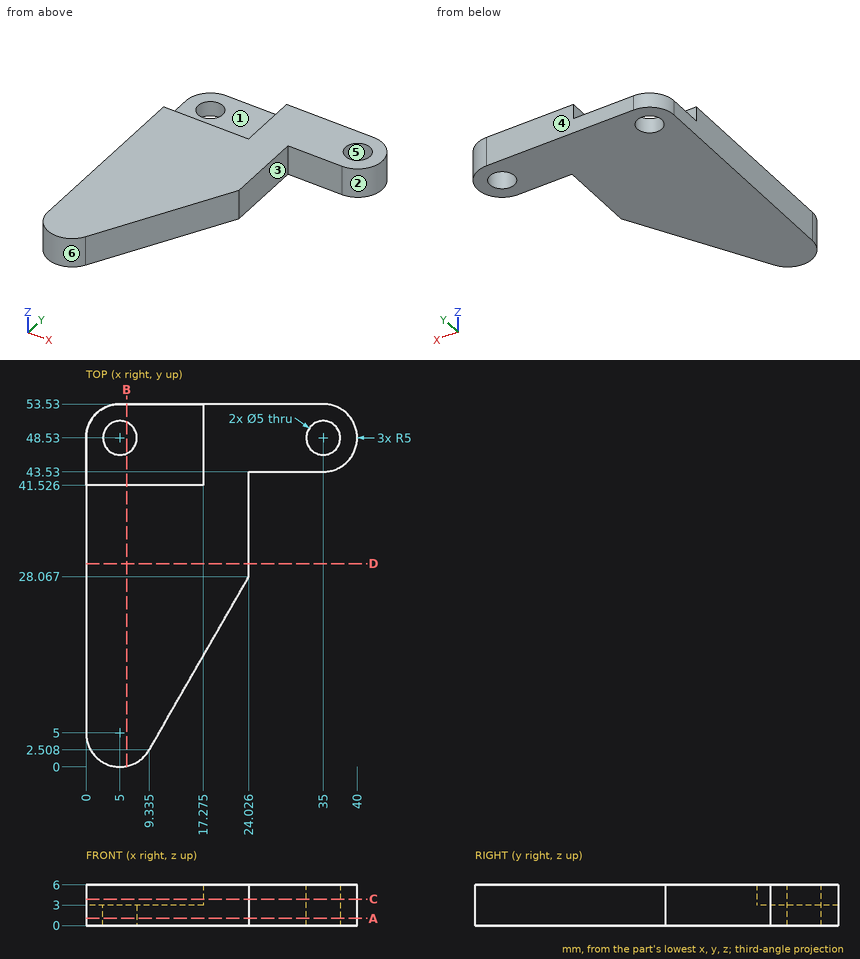
Input: dimensioned drawing with shaded views. Units: mm. Origin: part minimum x, y, z. A direction names the side the tool comes from. Round coordinates to 2 decimals unless told otherwise and drop trailing zeros. Loops run counter-clockwise (first coordinate to the right, second up) from the corner with the lowest first, then second, coordinate; pieces in that order, holes last.
1) Section query C-C on z = 3.9. Return the cut outline in (x, y) (1 decimal), plus the area to 3 significant figures.
Ans:
outline: (0, 5) arc R5 ccw to (9.3, 2.5) - (24, 28.1) - (24, 43.5) - (35, 43.5) arc R5 ccw to (35, 53.5) - (17.3, 53.5) - (17.3, 41.5) - (0, 41.5) - close; hole circle Ø5 at (35, 48.5)
area: 975 mm2
2) Pin query (flat end, axial travel): pin 1 (3.5 mm diameter, centred on x = 8, z = 4.5, fed in from +Y); pin 2 (1.5 mm diameter, centred on y = 45.5, z = 4, fed in from -X) (1 decimal); pin 3 (3.5 mm diameter, centred on x = 13, y = 50.5, fed in from +Z); pin 4 (2 mm diameter, centred on x = 14.5, z = 1, fed in from -Y) (1 decimal). Return the tip coordinate at first contact, or that it passes through.
Ans:
pin 1: stops at y = 53.53
pin 2: stops at x = 17.3
pin 3: stops at z = 3
pin 4: stops at y = 9.8
3) Section query A-A on z = 1.05. Return the cut outline in (x, y) (1 decimal).
Ans:
outline: (0, 5) arc R5 ccw to (9.3, 2.5) - (24, 28.1) - (24, 43.5) - (35, 43.5) arc R5 ccw to (35, 53.5) - (5, 53.5) arc R5 ccw to (0, 48.5) - close; hole circle Ø5 at (5, 48.5); hole circle Ø5 at (35, 48.5)
4) Set-up query: the marked faces 1, 2 and 3. Return all of +Z, -Z, +X, -X, +Y, -Y with unobstructed straight access to the full face (end or side cutting, diameter ignored); none if empty.
Ans:
face 1: +Z, -X, +Y
face 2: +Z, -Z, +X
face 3: +Z, -Z, +X, -Y
5) Section query B-B on x = 6. Return the cut outline in (y, z), plus the area to 3 significant figures.
Ans:
outline: (0.1, 0) - (46.24, 0) - (46.24, 3) - (41.53, 3) - (41.53, 6) - (0.1, 6) - close; (50.82, 0) - (53.53, 0) - (53.53, 3) - (50.82, 3) - close
area: 271 mm2
6) Material intervals for line 1 (X direction, y = 48, z = 1.25); line 2 (Y direction, x = 34, z = 3.25); line 3 (Y direction, x = 6.5, z = 2.2), sorted ascending.
Ans:
line 1: x = 0 to 2.56, 7.44 to 32.56, 37.44 to 39.97
line 2: y = 43.53 to 46.24, 50.82 to 53.53
line 3: y = 0.23 to 46.53, 50.53 to 53.53
7) Pull-direction query (Y, two-part tool) for the marked faces 4, 5 and 6; classes: released by +Y, released by -Y, zero draft, split by the parting line, or undercut.
Ans:
face 4: released by +Y
face 5: undercut
face 6: released by -Y
8) Section query D-D on y = 30. Return the cut outline in (x, z).
Ans:
outline: (0, 0) - (24.03, 0) - (24.03, 6) - (0, 6) - close
